Source: CAD feature listing. Evaluate the final solid. Frame: model axes, mm. A direction names the side the tool comes from. Give positions to 0.01 mm unless a question says otherwise; leave off trailing zeros. Write each loop counter-clockwise with the first axis right and the second up, starting at its lowest first coordinate (ties: lowest second). Pieces come first, ordered by that corner, then holes. Notation, with made-up numbers: M -14,34 L 13,34 A25 cw 13,68 Z; hole C -5,41 d3. An arc over 180 degrees is marked long. Return JSON: item names as keys, results as strings.
```python
from build123d import *

# Parameters (mm, degrees)
EXTRUDE_THIN1_DEPTH = 38.1


with BuildPart() as part:
    # Sketch1 → Extrude-Thin1 (new body)
    with BuildSketch(Plane(origin=(0, 0, 0), x_dir=(1, 0, 0), z_dir=(0, 1, 0))):
        with BuildLine():
            Line((40.452514176, 707.631658817), (37.717075708, 710.367097284))
            ThreePointArc((37.717075708, 710.367097284), (0, 725.990021576), (-37.717075708, 710.367097284))
            Line((-37.717075708, 710.367097284), (-40.452514176, 707.631658817))
            ThreePointArc((-40.452514176, 707.631658817), (-67.656084524, 687.982343635), (-99.656821316, 677.878746672))
            ThreePointArc((-99.656821316, 677.878746672), (-484.484817732, 484.484817732), (-677.878746672, 99.656821316))
            ThreePointArc((-677.878746672, 99.656821316), (-687.982343635, 67.656084524), (-707.631658817, 40.452514176))
            Line((-707.631658817, 40.452514176), (-710.367097284, 37.717075708))
            ThreePointArc((-710.367097284, 37.717075708), (-725.990021576, 0), (-710.367097284, -37.717075708))
            Line((-710.367097284, -37.717075708), (-707.631658817, -40.452514176))
            ThreePointArc((-707.631658817, -40.452514176), (-687.982343635, -67.656084524), (-677.878746672, -99.656821316))
            ThreePointArc((-677.878746672, -99.656821316), (-484.484817732, -484.484817732), (-99.656821316, -677.878746672))
            ThreePointArc((-99.656821316, -677.878746672), (-67.656084524, -687.982343635), (-40.452514176, -707.631658817))
            Line((-40.452514176, -707.631658817), (-37.717075708, -710.367097284))
            ThreePointArc((-37.717075708, -710.367097284), (0, -725.990021576), (37.717075708, -710.367097284))
            Line((37.717075708, -710.367097284), (40.452514176, -707.631658817))
            ThreePointArc((40.452514176, -707.631658817), (67.656084524, -687.982343635), (99.656821316, -677.878746672))
            ThreePointArc((99.656821316, -677.878746672), (484.484817732, -484.484817732), (677.878746672, -99.656821316))
            ThreePointArc((677.878746672, -99.656821316), (687.982343635, -67.656084524), (707.631658817, -40.452514176))
            Line((707.631658817, -40.452514176), (710.367097284, -37.717075708))
            ThreePointArc((710.367097284, -37.717075708), (725.990021576, 0), (710.367097284, 37.717075708))
            Line((710.367097284, 37.717075708), (707.631658817, 40.452514176))
            ThreePointArc((707.631658817, 40.452514176), (687.982343635, 67.656084524), (677.878746672, 99.656821316))
            ThreePointArc((677.878746672, 99.656821316), (484.484817732, 484.484817732), (99.656821316, 677.878746672))
            ThreePointArc((99.656821316, 677.878746672), (67.656084524, 687.982343635), (40.452514176, 707.631658817))
        make_face()
        with BuildLine():
            Line((38.656462951, 705.835607593), (35.921024484, 708.57104606))
            ThreePointArc((35.921024484, 708.57104606), (0, 723.450021576), (-35.921024484, 708.57104606))
            Line((-35.921024484, 708.57104606), (-38.656462951, 705.835607593))
            ThreePointArc((-38.656462951, 705.835607593), (-66.515541019, 685.712814936), (-99.287379903, 675.365757806))
            ThreePointArc((-99.287379903, 675.365757806), (-482.688766507, 482.688766507), (-675.365757806, 99.287379903))
            ThreePointArc((-675.365757806, 99.287379903), (-685.712814936, 66.515541019), (-705.835607593, 38.656462951))
            Line((-705.835607593, 38.656462951), (-708.57104606, 35.921024484))
            ThreePointArc((-708.57104606, 35.921024484), (-723.450021576, 0), (-708.57104606, -35.921024484))
            Line((-708.57104606, -35.921024484), (-705.835607593, -38.656462951))
            ThreePointArc((-705.835607593, -38.656462951), (-685.712814936, -66.515541019), (-675.365757806, -99.287379903))
            ThreePointArc((-675.365757806, -99.287379903), (-482.688766507, -482.688766507), (-99.287379903, -675.365757806))
            ThreePointArc((-99.287379903, -675.365757806), (-66.515541019, -685.712814936), (-38.656462951, -705.835607593))
            Line((-38.656462951, -705.835607593), (-35.921024484, -708.57104606))
            ThreePointArc((-35.921024484, -708.57104606), (0, -723.450021576), (35.921024484, -708.57104606))
            Line((35.921024484, -708.57104606), (38.656462951, -705.835607593))
            ThreePointArc((38.656462951, -705.835607593), (66.515541019, -685.712814936), (99.287379903, -675.365757806))
            ThreePointArc((99.287379903, -675.365757806), (482.688766507, -482.688766507), (675.365757806, -99.287379903))
            ThreePointArc((675.365757806, -99.287379903), (685.712814936, -66.515541019), (705.835607593, -38.656462951))
            Line((705.835607593, -38.656462951), (708.57104606, -35.921024484))
            ThreePointArc((708.57104606, -35.921024484), (723.450021576, 0), (708.57104606, 35.921024484))
            Line((708.57104606, 35.921024484), (705.835607593, 38.656462951))
            ThreePointArc((705.835607593, 38.656462951), (685.712814936, 66.515541019), (675.365757806, 99.287379903))
            ThreePointArc((675.365757806, 99.287379903), (482.688766507, 482.688766507), (99.287379903, 675.365757806))
            ThreePointArc((99.287379903, 675.365757806), (66.515541019, 685.712814936), (38.656462951, 705.835607593))
        make_face(mode=Mode.SUBTRACT)
    extrude(amount=EXTRUDE_THIN1_DEPTH)


solid = part.part
```
1) Line query: line 1 (Z direction, x = -594.5, y = 18.5); line 2 (Z direction, x = -220.5, y = 14); line 3 (X direction, y = 27, z = -140). Output: solid intervals per line, ascending. Write a range as [from, to].
Numbers:
{"line 1": "z = [-340.62, -335.48], [335.48, 340.62]", "line 2": "z = [-648.71, -646.03], [646.03, 648.71]", "line 3": "x = [-670.71, -668.11], [668.11, 670.71]"}
2) Contact query for flat-ended pins moving along their axis: pin 1 Ø10 at (x, y) = (151.5, 16.5) entering from +Z; pin 2 Ø1.5 at (x, y) = (-208.5, 30) entering from -Z; pin 3 Ø3 at (y, z) = (19.5, 314.5) entering from -X. Output: stop coordinate, or through.
Numbers:
{"pin 1": "stops at z = 669.32", "pin 2": "stops at z = -652.91", "pin 3": "stops at x = -609.49"}
3) Cut plane B-B, the plane z = -399.5. Return the cut outline in (x, y).
Numbers:
{"outline": "M -556.64,0 L -553.51,0 L -553.51,38.1 L -556.64,38.1 Z; M 553.51,0 L 556.64,0 L 556.64,38.1 L 553.51,38.1 Z"}
4) Set-up query: faces 4 (the face through (-0.559, 18.783, 723.447)), 5 (the face through (-488.8, 18.78, 480.13)). Return all of +Z, -Z, +X, -X, +Y, -Y with unobstructed straight access to the full face (end or side cutting, diameter ignored); none if empty.
Numbers:
{"face 4": "+Y, -Y", "face 5": "+Z, -X, +Y, -Y"}
5) Draft query along X for faces 1 (the face through (-687.77, 18.78, -68.08)), 2 (the face through (-66.948, 18.783, 685.497)), 3 (the face through (488.8, 18.78, -480.13)). Return one class per face: released by +X, released by -X, zero draft, split by the parting line, or undercut.
Numbers:
{"face 1": "released by -X", "face 2": "undercut", "face 3": "released by +X"}
